Verification items for the finished model (mm, model axes). A direction names the side the tool comes from. Coordinates: 2 decimals unless noted, no trailing zeros. Write each loop counter-clockwise with the first axis right and the second up, starting at its lowest first coordinate (ties: lowest second). Pieces come first, ordered by that corner, then holes. Notation, with made-up numbers: (39, 68) -> (59, 68) arc R20 cw to (59, 104) -> close; hole circle Ø2 at (87.5, 34.25). An arc over 180 degrees is marked (long way). Use CSV: the item, a comma, the result in double quotes.
```python
from build123d import *
from build123d.topology import SkipClean

# Parameters (mm, degrees)
SALIENTE_EXTRUIR1_DEPTH = 16
CROQUIS2_R              = 3.1
CORTAR_EXTRUIR1_DEPTH   = 500
CROQUIS3_R              = 9
CROQUIS3_R_2            = 3.1
SALIENTE_EXTRUIR2_DEPTH = 8
CORTAR_EXTRUIR2_DEPTH   = 4
CROQUIS7_R              = 9
SALIENTE_EXTRUIR3_DEPTH = 8
SALIENTE_EXTRUIR4_DEPTH = 1.6
CROQUIS9_R              = 3
CORTAR_EXTRUIR3_DEPTH   = 10
CORTAR_EXTRUIR4_START   = -8
CORTAR_EXTRUIR4_DEPTH   = 8
CORTAR_EXTRUIR6_START   = -8
CORTAR_EXTRUIR6_DEPTH   = 8


# Read off the part's stored shape, not the designer's step: Cortar-Extruir4, Cortar-Extruir6
with BuildPart() as part:
    # Croquis1 → Saliente-Extruir1 (new body)
    with BuildSketch(Plane(origin=(0, 0, 0), x_dir=(1, 0, 0), z_dir=(0, 1, 0))):
        with BuildLine():
            Line((-18.041618553, 2.75), (-56.041618553, 2.75))
            Line((-56.041618553, 2.75), (-56.041618553, 10.75))
            Line((-56.041618553, 10.75), (-14.747881204, 10.75))
            ThreePointArc((-14.747881204, 10.75), (18.25, 0), (-14.747881204, -10.75))
            Line((-14.747881204, -10.75), (-36.041618553, -10.75))
            Line((-36.041618553, -10.75), (-36.041618553, -2.75))
            Line((-36.041618553, -2.75), (-18.041618553, -2.75))
            Line((-18.041618553, -2.75), (-16.522711642, -2.75))
            ThreePointArc((-16.522711642, -2.75), (16.75, 0), (-16.522711642, 2.75))
            Line((-16.522711642, 2.75), (-18.041618553, 2.75))
        make_face()
    extrude(amount=SALIENTE_EXTRUIR1_DEPTH)

    # Croquis2 → Cortar-Extruir1 (cut)
    with BuildSketch(Plane.XY.offset(10.75)):
        with Locations((-27.041618553, 8)):
            Circle(CROQUIS2_R)
    extrude(amount=-CORTAR_EXTRUIR1_DEPTH, mode=Mode.SUBTRACT)

    # Croquis3 → Saliente-Extruir2 (add)
    with BuildSketch(Plane.XY.offset(10.75)):
        with Locations((-27.041618553, 8)):
            Circle(CROQUIS3_R)
        with Locations((-27.041618553, 8)):
            Circle(CROQUIS3_R_2, mode=Mode.SUBTRACT)
    extrude(amount=-SALIENTE_EXTRUIR2_DEPTH)

    # Croquis5 → Cortar-Extruir2 (cut)
    with BuildSketch(Plane.XY.offset(10.75)):
        Polygon((-27.041618553, 2.2), (-22.018671211, 5.1), (-22.018671211, 10.9), (-27.041618553, 13.8), (-32.064565895, 10.9), (-32.064565895, 5.1), align=None)
    extrude(amount=-CORTAR_EXTRUIR2_DEPTH, mode=Mode.SUBTRACT)

    # Croquis7 → Saliente-Extruir3 (add)
    with BuildSketch(Plane.XY.offset(-2.75)):
        with Locations((-47.041618553, 8)):
            Circle(CROQUIS7_R)
    extrude(amount=-SALIENTE_EXTRUIR3_DEPTH)

    # Croquis8 → Saliente-Extruir4 (add, symmetric)
    with SkipClean():  # the faces are left unmerged after this step: merging them gives an invalid solid
        with BuildSketch(Plane.XY.offset(-2.75)):
            with BuildLine():
                Line((-47.711899941, 13.459003834), (-48.138442643, 16.932915365))
                ThreePointArc((-48.138442643, 16.932915365), (-47.041618553, 17), (-45.944794462, 16.932915365))
                Line((-45.944794462, 16.932915365), (-46.371337164, 13.459003834))
                ThreePointArc((-46.371337164, 13.459003834), (-47.041618553, 13.5), (-47.711899941, 13.459003834))
            make_face()
            with BuildLine():
                Line((-43.731635925, 12.392495305), (-41.625283344, 15.18771959))
                ThreePointArc((-41.625283344, 15.18771959), (-42.541618553, 15.794228634), (-43.525038396, 16.284543681))
                Line((-43.525038396, 16.284543681), (-44.892597346, 13.062776694))
                ThreePointArc((-44.892597346, 13.062776694), (-44.291618553, 12.763139721), (-43.731635925, 12.392495305))
            make_face()
            with BuildLine():
                Line((-41.978841859, 10.149021207), (-38.757074872, 11.516580156))
                ThreePointArc((-38.757074872, 11.516580156), (-39.247389919, 12.5), (-39.853898962, 13.416335208))
                Line((-39.853898962, 13.416335208), (-42.649123247, 11.309982627))
                ThreePointArc((-42.649123247, 11.309982627), (-42.278478832, 10.75), (-41.978841859, 10.149021207))
            make_face()
            with BuildLine():
                Line((-41.582614719, 7.329718611), (-38.108703188, 6.903175909))
                ThreePointArc((-38.108703188, 6.903175909), (-38.041618553, 8), (-38.108703188, 9.096824091))
                Line((-38.108703188, 9.096824091), (-41.582614719, 8.670281389))
                ThreePointArc((-41.582614719, 8.670281389), (-41.541618553, 8), (-41.582614719, 7.329718611))
            make_face()
            with BuildLine():
                Line((-42.649123247, 4.690017373), (-39.853898962, 2.583664792))
                ThreePointArc((-39.853898962, 2.583664792), (-39.247389919, 3.5), (-38.757074872, 4.483419844))
                Line((-38.757074872, 4.483419844), (-41.978841859, 5.850978793))
                ThreePointArc((-41.978841859, 5.850978793), (-42.278478832, 5.25), (-42.649123247, 4.690017373))
            make_face()
            with BuildLine():
                Line((-44.892597346, 2.937223306), (-43.525038396, -0.284543681))
                ThreePointArc((-43.525038396, -0.284543681), (-42.541618553, 0.205771366), (-41.625283344, 0.81228041))
                Line((-41.625283344, 0.81228041), (-43.731635925, 3.607504695))
                ThreePointArc((-43.731635925, 3.607504695), (-44.291618553, 3.236860279), (-44.892597346, 2.937223306))
            make_face()
            with BuildLine():
                Line((-47.711899941, 2.540996166), (-48.138442643, -0.932915365))
                ThreePointArc((-48.138442643, -0.932915365), (-47.041618553, -1), (-45.944794462, -0.932915365))
                Line((-45.944794462, -0.932915365), (-46.371337164, 2.540996166))
                ThreePointArc((-46.371337164, 2.540996166), (-47.041618553, 2.5), (-47.711899941, 2.540996166))
            make_face()
            with BuildLine():
                Line((-50.35160118, 3.607504695), (-52.457953761, 0.81228041))
                ThreePointArc((-52.457953761, 0.81228041), (-51.541618553, 0.205771366), (-50.558198709, -0.284543681))
                Line((-50.558198709, -0.284543681), (-49.190639759, 2.937223306))
                ThreePointArc((-49.190639759, 2.937223306), (-49.791618553, 3.236860279), (-50.35160118, 3.607504695))
            make_face()
            with BuildLine():
                Line((-52.104395247, 5.850978793), (-55.326162234, 4.483419844))
                ThreePointArc((-55.326162234, 4.483419844), (-54.835847187, 3.5), (-54.229338143, 2.583664792))
                Line((-54.229338143, 2.583664792), (-51.434113858, 4.690017373))
                ThreePointArc((-51.434113858, 4.690017373), (-51.804758273, 5.25), (-52.104395247, 5.850978793))
            make_face()
            with BuildLine():
                Line((-52.500622387, 8.670281389), (-55.974533917, 9.096824091))
                ThreePointArc((-55.974533917, 9.096824091), (-56.041618553, 8), (-55.974533917, 6.903175909))
                Line((-55.974533917, 6.903175909), (-52.500622387, 7.329718611))
                ThreePointArc((-52.500622387, 7.329718611), (-52.541618553, 8), (-52.500622387, 8.670281389))
            make_face()
            with BuildLine():
                Line((-51.434113858, 11.309982627), (-54.229338143, 13.416335208))
                ThreePointArc((-54.229338143, 13.416335208), (-54.835847187, 12.5), (-55.326162234, 11.516580156))
                Line((-55.326162234, 11.516580156), (-52.104395247, 10.149021207))
                ThreePointArc((-52.104395247, 10.149021207), (-51.804758273, 10.75), (-51.434113858, 11.309982627))
            make_face()
            with BuildLine():
                Line((-49.190639759, 13.062776694), (-50.558198709, 16.284543681))
                ThreePointArc((-50.558198709, 16.284543681), (-51.541618553, 15.794228634), (-52.457953761, 15.18771959))
                Line((-52.457953761, 15.18771959), (-50.35160118, 12.392495305))
                ThreePointArc((-50.35160118, 12.392495305), (-49.791618553, 12.763139721), (-49.190639759, 13.062776694))
            make_face()
        extrude(amount=SALIENTE_EXTRUIR4_DEPTH, both=True)

    # Croquis9 → Cortar-Extruir3 (cut)
    with SkipClean():  # the faces are left unmerged after this step: merging them gives an invalid solid
        with BuildSketch(Plane.XY.offset(-2.75)):
            with Locations((-47.041618553, 8)):
                Circle(CROQUIS9_R)
        extrude(amount=-CORTAR_EXTRUIR3_DEPTH, mode=Mode.SUBTRACT)

    # Cortar-Extruir4 outline → Cortar-Extruir4 (cut)
    with SkipClean():  # the faces are left unmerged after this step: merging them gives an invalid solid
        with BuildSketch(Plane(origin=(0, 0, -10.75), x_dir=(-1, 0, 0), z_dir=(0, 0, -1)).offset(CORTAR_EXTRUIR4_START)):
            with BuildLine():
                Line((56.041618553, 16), (51.164724178, 16))
                ThreePointArc((51.164724178, 16), (54.726276991, 12.684658439), (56.041618553, 8))
                Line((56.041618553, 8), (56.041618553, 16))
            make_face()
            with BuildLine():
                Line((56.041618553, 0), (56.041618553, 8))
                ThreePointArc((56.041618553, 8), (54.726276991, 3.315341561), (51.164724178, 0))
                Line((51.164724178, 0), (56.041618553, 0))
            make_face()
        extrude(amount=CORTAR_EXTRUIR4_DEPTH, mode=Mode.SUBTRACT)

    # Cortar-Extruir6 outline → Cortar-Extruir6 (cut)
    with SkipClean():  # the faces are left unmerged after this step: merging them gives an invalid solid
        with BuildSketch(Plane.XY.offset(10.75).offset(CORTAR_EXTRUIR6_START)):
            with BuildLine():
                ThreePointArc((-31.164724178, 0), (-34.726276991, 3.315341561), (-36.041618553, 8))
                Line((-36.041618553, 8), (-36.041618553, 0))
                Line((-36.041618553, 0), (-31.164724178, 0))
            make_face()
            with BuildLine():
                ThreePointArc((-36.041618553, 8), (-34.726276991, 12.684658439), (-31.164724178, 16))
                Line((-31.164724178, 16), (-36.041618553, 16))
                Line((-36.041618553, 16), (-36.041618553, 8))
            make_face()
        extrude(amount=CORTAR_EXTRUIR6_DEPTH, mode=Mode.SUBTRACT)


solid = part.part
```
1) Cross-section at A-A (x = 0). Record the boundary of the cut face in (y, z), plus the area to 3 significant figures.
Return value:
outline,"(0, -18.25) -> (16, -18.25) -> (16, -16.75) -> (0, -16.75) -> close; (0, 16.75) -> (16, 16.75) -> (16, 18.25) -> (0, 18.25) -> close"
area,"48.0 mm2"
2) Cross-section at B-B (x = -18). Record the boundary of the cut face in (y, z), plus the area to 3 significant figures.
Return value:
outline,"(0, -10.75) -> (16, -10.75) -> (16, -2.75) -> (0, -2.75) -> close; (0, 2.75) -> (16, 2.75) -> (16, 10.75) -> (0, 10.75) -> close"
area,"256 mm2"
3) Gauge pin test, flat ends, axial feed: pin 1 (12 mm diameter, centred on x = -4.5, z = -14, fed in from +Y); pin 2 (1.5 mm diameter, centred on y = 5, z = -2.5, fed in from -X); pin 3 (9 mm diameter, centred on x = -26, y = 6, fed in from +Z). Record the tip position at first contact, or that the pin passes through.
Return value:
pin 1,"y = 16"
pin 2,"x = -55.74"
pin 3,"z = 10.75"
4) Scan lines: L1, parallel to Z at x = -24, y = 12.75; L2, parallel to X at y = 10.25, z = -2.5; L3, parallel to Y at x = -18, z = -8. Record each from-to range of solid material in increasing order.
Return value:
L1,"-10.75 to -2.75, 2.75 to 10.75"
L2,"-52.34 to -52.06, -42.02 to -41.74, 16.56 to 18.08"
L3,"0 to 16"
5) Set-up check for faces 4 (the flat face through (-44.22, 1.35, -1.96)), 5 (the flat face through (-24.565, 3.63, 8.778)), 6 (the flat face through (-51, 2, -1.15)): record each of +Z, -Z, +X, -X, +Y, -Y from which the full face is reachable in a straight line by a thin tool's end or side.
Return value:
face 4,"+Z, -Y"
face 5,"+Z"
face 6,"+Z, -X, +Y, -Y"
6) Mould release check, pull along Y, two halves, no side actions. Record for faces 1 (the flat face through (-47, 15, -1.15)), 2 (the flat face through (-22.019, 8, 9)), 3 (the flat face through (-49.884, 1.304, -1.961)): released by +Y, released by -Y, zero draft, split by the parting line, or undercut.
Return value:
face 1,"zero draft"
face 2,"undercut"
face 3,"released by -Y"
7) Cross-section at C-C (z = 0). Record the boundary of the cut face in (x, y).
Return value:
outline,"(16.75, 0) -> (18.25, 0) -> (18.25, 16) -> (16.75, 16) -> close"
